Autodesk Inventor part; units mm, degrees
ref_plane "YZ Plane" through (0, 0, 0) normal (1, 0, 0) x (0, 1, 0)
ref_plane "XZ Plane" through (0, 0, 0) normal (0, 1, 0) x (-1, 0, 0)
ref_plane "XY Plane" through (0, 0, 0) normal (0, 0, 1) x (1, 0, 0)
sketch "Sketch1" plane through (0, 0, 0) normal (0, 1, 0) x (-1, 0, 0)
  line L0 (0, 0) -> (6.35, 0)
  line L1 (6.35, 0) -> (6.35, -101.6)
  line L2 (6.35, -101.6) -> (0, -101.6)
  line L3 (0, -101.6) -> (0, 0)
  dimension "d0" = 6.35
  dimension "d1" = 101.6
extrude "Extrusion1" add sketch "Sketch1" along normal blind 101.6
sketch "Sketch2" plane through (0, 0, 0) normal (0, -1, 0) x (1, 0, 0)
  line L0 (0, 0) -> (0, -25.4)
  line L1 (0, 0) -> (0, -101.6)
  line L2 (0, -101.6) -> (0, -76.2)
  line L3 (0, -25.4) -> (-3.175, -25.4)
  line L4 (-3.175, -25.4) -> (-3.175, -12.7)
  line L5 (-3.175, -12.7) -> (0, -12.7)
  line L6 (0, -12.7) -> (0, -25.4)
  line L7 (0, -76.2) -> (-3.175, -76.2)
  line L8 (-3.175, -76.2) -> (-3.175, -88.9)
  line L9 (-3.175, -88.9) -> (0, -88.9)
  line L10 (0, -88.9) -> (0, -76.2)
  dimension "d4" = 25.4
  dimension "d5" = 25.4
  dimension "d6" = 3.175
  dimension "d7" = 12.7
  dimension "d8" = 3.175
  dimension "d9" = 12.7
extrude "Extrusion2" add sketch "Sketch2" along normal blind 12.7
sketch "Sketch3" plane through (0, 0, -101.6) normal (1, 0, 0) x (0, 0, -1)
  line L0 (0, 0) -> (0, 101.6)
  line L1 (0, 0) -> (-12.7, 0)
  line L2 (-101.6, 0) -> (-101.6, 101.6)
  line L3 (-95.25, 95.25) -> (-95.25, 6.35)
  line L4 (-95.25, 6.35) -> (-6.35, 6.35)
  line L5 (-6.35, 6.35) -> (-6.35, 95.25)
  line L6 (-6.35, 95.25) -> (-95.25, 95.25)
  line L7 (-101.6, 0) -> (0, 0)
  line L8 (0, 101.6) -> (-101.6, 101.6)
  dimension "d20" = 88.9
  dimension "d22" = 6.35
  dimension "d23" = 6.35
  dimension "d24" = 6.35
extrude "Extrusion4" add sketch "Sketch3" along normal blind 3.175 contours L6 L5 L4 L3
properties part number "top"
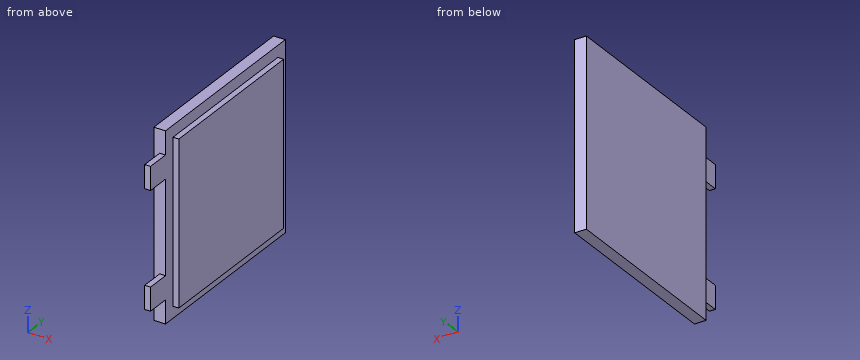
The model under review builds one solid part; all positions refer to its coordinate system, in mm. Round coordinates to 2 decimals unless told otherwise and drop trailing zeros. Order: outer loops, then holes, each group sorted by start corner. A loop starts at its lowest first (then second) coordinate and runs counter-clockwise, first axis right, second up. Notation, with made-up numbers: (85.25, 53) -> (144.25, 53) arc R21 cw to (144.25, 75) -> close; hole circle Ø7 at (-21.5, -6.75). An arc over 180 degrees is marked (long way). Use a Markdown table: item, result.
Q1. We need section C-C on x = -4.75. Write out the cut boundary in (y, z).
Values:
| item | result |
|---|---|
| outline | (0, -101.6) -> (101.6, -101.6) -> (101.6, 0) -> (0, 0) -> close |
Q2. For line 1 (Z direction, x = 1.25, y = 11); line 2 (Y direction, x = 1.5, z = -47.5); line 3 (Y direction, x = -3.25, z = -72), list the stretches that pass through material, from the lowest coordinate up.
Values:
| item | result |
|---|---|
| line 1 | z = -95.25 to -6.35 |
| line 2 | y = 6.35 to 95.25 |
| line 3 | y = 0 to 101.6 |
Q3. Clearance check with flat-ended pins moving along their axes: P1, Ø1.5, axis at x = 2, z = -62, coming from the +Y side; P2, Ø2, axis at x = 1.5, y = 68.5, coming from the +Z side; P3, Ø1.6, axis at x = 2.5, z = -59.5, coming from the -Y side. State where each tip first meets the part, or that it passes through.
Values:
| item | result |
|---|---|
| P1 | stops at y = 95.25 |
| P2 | stops at z = -6.35 |
| P3 | stops at y = 6.35 |
Q4. We need section B-B on y = 59. Write out the cut boundary in (x, z) (3 decimals).
Values:
| item | result |
|---|---|
| outline | (-6.35, -101.6) -> (0, -101.6) -> (0, -95.25) -> (3.175, -95.25) -> (3.175, -6.35) -> (0, -6.35) -> (0, 0) -> (-6.35, 0) -> close |
Q5. We need section A-A on z = -74. Write out the cut boundary in (x, y) (3 decimals), then the cut area to 3 significant figures.
Values:
| item | result |
|---|---|
| outline | (-6.35, 0) -> (0, 0) -> (0, 6.35) -> (3.175, 6.35) -> (3.175, 95.25) -> (0, 95.25) -> (0, 101.6) -> (-6.35, 101.6) -> close |
| area | 927 mm^2 |
